```python
from build123d import *

# Parameters (mm, degrees)
BLANKSKE_W            = 67
BLANKSKE_H            = 5.125
BLANK_DEPTH           = 5
TOOTHCUTSIM_DEPTH     = 68.381493194
TEETHCUTS_COUNT       = 20
TEETHCUTS_PITCH       = 3.534291731
CROQUIS1_W            = 67
CROQUIS1_H            = 1.296875
CORTAR_EXTRUIR1_DEPTH = 10


with BuildPart() as part:
    # BlankSke → Blank (new body)
    with BuildSketch(Plane.XY):
        with Locations((33.5, 2.5625)):
            Rectangle(BLANKSKE_W, BLANKSKE_H)
    extrude(amount=-BLANK_DEPTH)

    # TooCutSkeSim → ToothCutSim (cut, through all)
    with BuildSketch(Plane.XY):
        Polygon((0.645891955, 2.59375), (-0.645891955, 2.59375), (-1.307086602, 5.1504), (1.307086602, 5.1504), align=None)
    toothcutsim = extrude(amount=-TOOTHCUTSIM_DEPTH, mode=Mode.SUBTRACT)

    # TeethCuts: ToothCutSim ×20
    with Locations(*[(i * TEETHCUTS_PITCH, 0, 0) for i in range(1, TEETHCUTS_COUNT)]):
        add(toothcutsim, mode=Mode.SUBTRACT)

    # Croquis1 → Cortar-Extruir1 (cut)
    with BuildSketch(Plane.XY):
        with Locations((33.5, 0.6484375)):
            Rectangle(CROQUIS1_W, CROQUIS1_H)
    extrude(amount=-CORTAR_EXTRUIR1_DEPTH, mode=Mode.SUBTRACT)


solid = part.part
```
Design review of the part built by this model. Coordinates are the model's own, in mm. A direction names the side the tool comes from. Coordinates: 2 decimals unless noted, no trailing zeros. Order: outer loops, then holes, each group sorted by start corner. A loop starts at its lowest first (then second) coordinate and runs counter-clockwise, first axis right, second up.
1) Take a section at A-A, the plane x = 10.5. Give the boundary of the cut face in (y, z), and give its area (3 significant figures).
2) Mouldability with a two-part tool opening along X and no side actions: class faces 1 (the flat face through (4, 2.594, -2)), 2 (the flat face through (66.183, 3.842, -2.465)), 3 (the flat face through (0.98, 3.88, -2.46)) as +X half, -X half, draft (parallel to the pull), parting line (faces both ways), or undercut.
3) Clearance check with a flat-ended pin moving along its axis: pin 1 (1 mm diameter, centred on x = 10.5, z = -3.5, fed in from +Y). State where the tip first meets the part, or that it passes through.
4) For faces 4 (the flat face through (46.924, 3.877, -2.465)), 5 (the flat face through (67, 2, -2)), list the 3-axis set-ups (+Z, -Z, +X, -X, +Y, -Y) from which the entire face can be reached by the end or side of a thin tool; tool diameter is ignored.
5) Take a section at B-B, the plane y = 4.45. State how many separate pieces and enclosed holes the cut face has, and give its area (3 significant figures).
6) Wall thickness on line 1 along Y through (x, z) = (39, -1.4): over which ranges is the line inside the solid? List them lowest first.
Returned:
1. outline: (1.3, -5) - (2.59, -5) - (2.59, 0) - (1.3, 0) - close
1. area: 6.48 mm2
2. face 1: undercut
2. face 2: +X half
2. face 3: -X half
3. pin 1: stops at y = 2.59
4. face 4: +Z, -Z, +Y
4. face 5: +Z, -Z, +X, +Y, -Y
5. separate pieces: 19
5. enclosed holes: 0
5. area: 122 mm2
6. line 1: y = 1.3 to 2.59
